CAD build for the part. Positions are in the model's coordinates, mm. Face numbers are marked on the shaded views. A direction names the side the tool comes from. Give positions to 0.01 mm unless a question says otherwise; leave off trailing zeros. Loops run counter-clockwise (first coordinate to the right, second up) from the corner with the lowest first, then second, coordinate; pieces in that order, holes last. Notation, with made-up numbers: (10, 24.25) - (35, 24.25) arc R8 ccw to (35, 36.25) - close; hole circle Ø8 at (13.25, -8.5). An arc over 180 degrees is marked (long way). Return JSON: item names as keys, results as strings.
from build123d import *

# Parameters (mm, degrees)
SKETCH3_R         = 1.5
EXTRUDE1_DEPTH    = 12
CHAMFER1_SIZE     = 0.3
SKETCH4_OUTSIDE_W = 12.89
SKETCH4_OUTSIDE_H = 12.89
EXTRUDE2_DEPTH    = 26.24


with BuildPart() as part:
    # Sketch2 → Revolve3 (revolve)
    with BuildSketch(Plane.XY):
        Polygon((0, 0), (-1.5, 0), (-1.5, 3), (-2.8, 3), (-2.8, 25.24), (0, 25.24), align=None)
    revolve(axis=Axis((0, 33.398198685, 0), (0, -1, 0)))

    # Sketch3 → Extrude1 (cut)
    with BuildSketch(Plane(origin=(0, 25.24, 0), x_dir=(1, 0, 0), z_dir=(0, 1, 0))):
        Circle(SKETCH3_R)
    extrude(amount=-EXTRUDE1_DEPTH, mode=Mode.SUBTRACT)

    # Chamfer1
    chamfer1_edges = [part.edges().sort_by_distance(p)[0] for p in [
        (-1.5, 25.24, 0),
        (2.8, 25.24, 0),
        (2.8, 3, 0),
    ]]
    chamfer(chamfer1_edges, length=CHAMFER1_SIZE)

    # Sketch4 outside → Extrude2 (cut, through all)
    with BuildSketch(Plane(origin=(0, 25.24, 0), x_dir=(1, 0, 0), z_dir=(0, 1, 0))):
        Rectangle(SKETCH4_OUTSIDE_W, SKETCH4_OUTSIDE_H)
        Polygon((2.829016319, 0), (1.41450816, 2.45), (-1.41450816, 2.45), (-2.829016319, 0), (-1.41450816, -2.45), (1.41450816, -2.45), align=None, mode=Mode.SUBTRACT)
    extrude(amount=-EXTRUDE2_DEPTH, mode=Mode.SUBTRACT)


solid = part.part
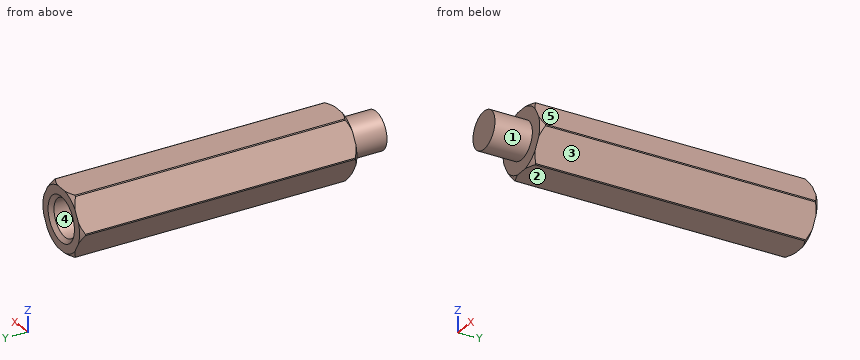
1. Cut at C-C, the plane x = 2.1. Write the cut outline in (y, z), plus the area to 3 significant figures.
Values follow:
{"outline": "(3, -1.26) - (25.24, -1.26) - (25.24, 1.26) - (3, 1.26) - close", "area": "56.2 mm²"}
2. Pull direction Z, two halves, no side cores. Call the marked faces 3, 4 and 5: +Z half, -Z half, draft (parallel to the pull), parting line (faces both ways), or undercut.
Values follow:
{"face 3": "-Z half", "face 4": "undercut", "face 5": "+Z half"}
3. Drop flat-ended pins along their axis: P1, Ø2.5, axis at x = 0, z = 0, coming from the -Y side; P2, Ø2, axis at y = 6.5, z = 2, coming from the -X side. Give the stop position or say it passes through.
Values follow:
{"P1": "stops at y = 0", "P2": "stops at x = -2.25"}
4. Cut at B-B, the plane x = 0. Write the cut outline in (y, z), plus the area to 3 significant figures.
Values follow:
{"outline": "(0, -1.5) - (3, -1.5) - (3, -2.45) - (25.24, -2.45) - (25.24, -1.8) - (24.94, -1.5) - (13.24, -1.5) - (13.24, 1.5) - (24.94, 1.5) - (25.24, 1.8) - (25.24, 2.45) - (3, 2.45) - (3, 1.5) - (0, 1.5) - close", "area": "81.9 mm²"}
5. Drill centre lines: probe 1 along Z at (x, y) = (0.65, 21.5); probe 2 along X at (y, z) = (22.25, 0); probe 3 along X at (y, z) = (19.25, -1.15). Where is each one in solid material? Low to high.
Values follow:
{"probe 1": "z = -2.45 to -1.35, 1.35 to 2.45", "probe 2": "x = -2.8 to -1.5, 1.5 to 2.8", "probe 3": "x = -2.17 to -0.96, 0.96 to 2.17"}
6. Which spindle directions (+Z, -Z, +X, -X, +Y, -Y) get a long thin tool onto all of the face, cutting with end or side? Do the marked faces 1 and 2. Say none if no direction does.
Values follow:
{"face 1": "-Y", "face 2": "-Z, +X, -X, +Y, -Y"}
7. Cut at A-A, the plane y = 17.25. Write the cut outline in (x, z).
Values follow:
{"outline": "(-2.8, -0.05) - (-1.44, -2.4) arc R2.8 ccw to (-1.36, -2.45) - (1.36, -2.45) arc R2.8 ccw to (1.44, -2.4) - (2.8, -0.05) arc R2.8 ccw to (2.8, 0.05) - (1.44, 2.4) arc R2.8 ccw to (1.36, 2.45) - (-1.36, 2.45) arc R2.8 ccw to (-1.44, 2.4) - (-2.8, 0.05) arc R2.8 ccw to start; hole circle Ø3 at (0, 0)"}
